Input: part model. Units: mm. Frame: model coordinates. Face numbers are marked on the shaded views. Give positions to 0.01 mm unless a question says otherwise; leave off trailing zeros. Loops run counter-clockwise (first coordinate to the right, second up) from the corner with the lowest first, then second, coordinate; pieces in that order, holes last. Notation, with made-up numbers: (35, 72) -> (81, 72) arc R31 cw to (81, 103) -> close; hole circle Ø5 at (73, 74). An arc over 180 degrees is marked (long way). One line per question, with ' | ' between items.
Autodesk Inventor part; units mm, degrees
ref_plane "Work Plane8" through (0, 0, 20) normal (0, 0, 1) x (1, 0, 0)
ref_plane "YZ Plane" through (0, 0, 0) normal (1, 0, 0) x (0, 1, 0)
ref_plane "XZ Plane" through (0, 0, 0) normal (0, 1, 0) x (-1, 0, 0)
sketch "Sketch1" plane through (0, 0, 0) normal (0, 0, 1) x (1, 0, 0)
  circle A0 centre (0, 0) radius 59.2469 construction
  line L0 (0, 0) -> (59.2469, 0)
  line L1 (0, 0) -> (59.2469, 4.025)
  line L2 (59.2469, 0) -> (59.2469, 4.025)
  circle A1 centre (0, 0) radius 75
  point P0 (56.8, 0)
  dimension "d56" = 59.2469
  dimension "d57" = 4.025
  dimension "d400" = 75
  dimension "d495" = 2.5
  dimension "d496" = 8
  dimension "d531" = 5.5
  dimension "d532" = 5.5
  dimension "d533" = 5.5
  dimension "d537" = 24.5
  dimension "d538" = 3
  dimension "d543" = 5.5
  dimension "d549" = 3
  dimension "d550" = 3
  dimension "d567" = 5.5
  dimension "d568" = 5.5
sketch "Sketch7" plane through (0, 0, 0) normal (0, 1, 0) x (-1, 0, 0)
  line L0 (0, 0) -> (0, 61.9844)
  line L1 (0, 0) -> (-59.2469, 0) construction
  line L2 (0, 61.9844) -> (-59.2469, 0) construction
  line L3 (0, 61.9844) -> (-64.8494, 0) construction
  line L4 (0, 61.9844) -> (-58.9939, -5.5968) construction
  line L5 (0, 0) -> (0, -61.9844)
  line L6 (0, -61.9844) -> (-59.2469, 0) construction
  line L7 (0, -61.9844) -> (-64.8494, 0) construction
  line L8 (0, -61.9844) -> (-58.9939, 5.5968) construction
  line L9 (-58.9939, 5.5968) -> (-64.8494, 0) construction
  line L10 (-54.1083, 0) -> (-62.8579, -8.363) construction
  line L11 (-54.1083, 0) -> (-38.773, -14.6579) construction
  line L12 (0, -94.3812) -> (0, 132.3969)
  line L13 (-75, -5.9919) -> (-75, 6.008)
  line L14 (105, 0) -> (-105, 0)
  line L15 (-62.0481, 2.6775) -> (-56.4456, -2.6775) construction
  line L16 (-56.4456, 2.6775) -> (-62.0481, -2.6775) construction
  line L17 (-26.151, -15.9303) -> (-40.3783, -15.9303) construction
  line L18 (-40.3783, -15.9303) -> (-40.3783, -12.7539) construction
  line L19 (-40.3783, -12.7539) -> (-26.151, -12.7539) construction
  line L20 (-26.151, -12.7539) -> (-26.151, -15.9303) construction
  point P0 (-75, 0)
  dimension "Roller_Side_difference" = -0.0002
  dimension "d90" = 61.9844
  dimension "d201" = 75
  dimension "d343" = 92.587
  dimension "d344" = 92.588
  dimension "d367" = 8.1
sketch "Roller1" plane through (0, 0, 0) normal (0, 1, 0) x (-1, 0, 0)
  line L0 (0, 61.9844) -> (-58.9939, -5.5968) construction
  line L1 (0, 61.9844) -> (-64.8494, 0) construction
  line L2 (-54.1083, 0) -> (-38.773, -14.6579) construction
  line L3 (0, -61.9844) -> (-64.8494, 0) construction
  line L4 (-54.0606, 0.0927) -> (-58.9462, -5.5041)
  line L5 (-58.9462, -5.5041) -> (-64.7589, 0.0519)
  line L6 (-64.7589, 0.0519) -> (-59.3884, 5.1851)
  line L7 (-59.3884, 5.1851) -> (-54.0606, 0.0927)
  line L8 (-56.0019, 1.9482) -> (-61.1299, -3.4168)
  line L9 (-61.8526, -2.7261) -> (-56.7246, 2.639)
  point P0 (0, 0)
  dimension "d345" = 0.025
  dimension "d346" = 0.025
  dimension "d347" = 0.1
  dimension "d348" = 0.1
  dimension "d349" = 272.588
  dimension "d350" = 272.587
  dimension "d617" = 0.9997
sketch "Roller2" plane through (0, 0, 0) normal (0, 1, 0) x (-1, 0, 0)
  line L0 (0, -61.9844) -> (-58.9939, 5.5968) construction
  line L1 (-54.1083, 0) -> (-62.8579, -8.363) construction
  line L2 (0, -61.9844) -> (-64.8494, 0) construction
  line L3 (0, 61.9844) -> (-64.8494, 0) construction
  line L4 (-58.9956, 5.5606) -> (-54.1429, 0.0016)
  line L5 (-54.1429, 0.0016) -> (-59.4789, -5.0987)
  line L6 (-59.4789, -5.0987) -> (-64.8132, 0)
  line L7 (-64.8132, 0) -> (-58.9956, 5.5606)
  line L8 (-61.9044, 2.7803) -> (-56.8109, -2.5486)
  line L9 (-61.1815, 3.4713) -> (-56.088, -1.8576)
  point P0 (0, 0)
  dimension "d351" = 0.025
  dimension "d352" = 0.025
  dimension "d354" = 0.025
  dimension "d355" = 92.587
  dimension "d356" = 92.588
  dimension "d370" = 0.025
  dimension "d371" = 1
sketch "Sketch22" plane through (0, 0, 0) normal (0, 1, 0) x (-1, 0, 0)
  line L0 (-31.756, 8.0215) -> (-17.5287, 8.0215) construction
  line L1 (-17.5287, 8.0215) -> (-17.5287, 4.8451) construction
  line L2 (-17.5287, 4.8451) -> (-31.756, 4.8451) construction
  line L3 (-31.756, 4.8451) -> (-31.756, 8.0215) construction
  point P0 (0, 0)
  dimension "Roller_Side_difference" = -0.0002
sketch "Sketch2" plane through (0, 0, 0) normal (0, 1, 0) x (-1, 0, 0)
  line L0 (0, 0) -> (0, 59.2469) construction
  line L1 (0, 0) -> (-59.2469, 0)
  line L2 (0, 0) -> (0, -59.2469)
  line L3 (0, -59.2469) -> (-59.2469, 0) construction
  line L4 (0, 59.2469) -> (-59.2469, 0) construction
  line L5 (-50.4879, 53.555) -> (0, 59.2469) construction
  line L6 (-29.7354, 7.189) -> (0, 59.2469) construction
  line L7 (-29.7354, 7.189) -> (0, -59.2469) construction
  line L8 (-48.8381, -26.254) -> (0, -59.2469) construction
  point P0 (-40.4258, 18.8211)
sketch "Sketch23" plane through (0, 0, 0) normal (0, 1, 0) x (-1, 0, 0)
  line L0 (0, -61.9844) -> (-58.9939, 5.5968) construction
  line L1 (0, -61.9844) -> (-64.8494, 0) construction
  line L2 (0, 61.9844) -> (-58.9939, -5.5968) construction
  line L3 (-58.9939, 5.5968) -> (-64.8494, 0) construction
  line L4 (0, 61.9844) -> (-64.8494, 0) construction
  line L5 (-58.9939, 5.5968) -> (-58.9939, -5.5968) construction
  line L6 (105, 0) -> (-105, 0)
  line L7 (-57.6514, 4.0968) -> (-54.1326, 0.0658)
  line L8 (-54.1326, -0.0658) -> (-57.6514, -4.0968)
  line L9 (-60.5995, 4.0968) -> (-64.81, 0.0723)
  line L10 (-64.81, -0.0723) -> (-60.5995, -4.0968)
  arc A0 (-64.81, 0.0723) -> (-64.81, -0.0723) centre (-64.7409, 0) ccw
  arc A1 (-54.1326, -0.0658) -> (-54.1326, 0.0658) centre (-54.2079, 0) ccw
  line L11 (-57.6514, 4.0968) -> (-57.6514, 5.5968)
  line L12 (-57.6514, 5.5968) -> (-25, 5.5968)
  line L13 (-25, 5.5968) -> (-25, -5.5968)
  line L14 (-25, -5.5968) -> (-57.6514, -5.5968)
  line L15 (-57.6514, -5.5968) -> (-57.6514, -4.0968)
  line L16 (-60.5995, 4.0968) -> (-60.5995, 5.5968)
  line L17 (-60.5995, 5.5968) -> (-75, 5.5968)
  line L18 (-75, 5.5968) -> (-75, -5.5968)
  line L19 (-60.5995, -4.0968) -> (-60.5995, -5.5968)
  line L20 (-60.5995, -5.5968) -> (-75, -5.5968)
  line L21 (-58.9939, 5.5968) -> (-58.9939, 5.5968)
  line L22 (-58.9939, -5.5968) -> (-58.9939, -5.5968)
  line L23 (0, -94.3812) -> (0, 132.3969)
  line L24 (-64.8856, 0) -> (-75, 0)
  point P0 (0, 0)
  point P1 (-54.0752, 0)
  point P2 (-64.8409, 0)
  point P3 (-75, 0)
  dimension "d378" = 90
  dimension "d379" = 0.1
  dimension "d380" = 0.025
  dimension "d381" = 0.025
  dimension "d382" = 0.025
  dimension "d383" = 0.025
  dimension "d384" = 11.1935
  dimension "d385" = 0
  dimension "d386" = 0
  dimension "d391" = 25
  dimension "d392" = 75
  dimension "d393" = 1.5
  dimension "d394" = 1.5
  dimension "d395" = 1.5
  dimension "d396" = 1.5
revolve "RevRoller1" [suppressed]
fillet "Fillet1" [suppressed]
sketch "Sketch48" plane through (56.7246, 0, 2.639) normal (-0.691, 0, 0.7229) x (0.7229, 0, 0.691)
  line L0 (-2.5, 0.25) -> (2.5, 0.25)
  line L1 (2.5, 0.25) -> (2.5, -0.25)
  line L2 (2.5, -0.25) -> (-2.5, -0.25)
  line L3 (-2.5, -0.25) -> (-2.5, 0.25)
  line L4 (-2.5, 0.25) -> (2.5, -0.25) construction
  line L5 (2.5, 0.25) -> (-2.5, -0.25) construction
  line L6 (-0.25, -2.5) -> (0.25, -2.5)
  line L7 (0.25, -2.5) -> (0.25, 2.5)
  line L8 (0.25, 2.5) -> (-0.25, 2.5)
  line L9 (-0.25, 2.5) -> (-0.25, -2.5)
  line L10 (-0.25, -2.5) -> (0.25, 2.5) construction
  line L11 (0.25, -2.5) -> (-0.25, 2.5) construction
  point P0 (-42.8293, 0)
  point P1 (0, 0)
  point P2 (-0.25, 0.25)
  point P3 (-0.25, -0.25)
  point P4 (0.25, -0.25)
  point P5 (0.25, 0.25)
  dimension "d621" = 5
  dimension "d622" = 0.5
  dimension "d623" = 0.5
  dimension "d624" = 5
extrude "Extrusion39" [suppressed]
sketch "Sketch40" plane through (0, 0, -5.231) normal (0, 0, -1) x (-1, 0, 0)
  circle A0 centre (53.5, 0) radius 2.75
  circle A1 centre (0, 0) radius 53.5
  point P0 (53.4293, 2.7491)
  point P1 (53.4293, -2.7491)
  dimension "d585" = 8
  dimension "d587" = 1.75
  dimension "d589" = 3
  dimension "d592" = 2
  dimension "d593" = 12
  dimension "d594" = 12
  dimension "d611" = 360
pattern_circular "Circular Pattern13" [suppressed]
feature "Move Body7" [suppressed]
revolve "Revolution13" [suppressed]
fillet "Fillet3" [suppressed]
pattern_circular "Circular Pattern14" [suppressed]
feature "Move Body6" [suppressed]
revolve "Revolution14" add sketch "Sketch23" angle 360 about axis through (0, 0, -10) along (0, 0, 1) contours A1 L7 L11 L12 L13 L6 | L6 L13 L14 L15 L8 A1
revolve "OuterRim_Top2" [suppressed]
revolve "OuterRim_Bottom2" [suppressed]
ref_plane "Work Plane8" through (0, 0, 20) normal (0, 0, 1) x (1, 0, 0)
sketch "Sketch49" plane through (0, 0, 20) normal (0, 0, 1) x (1, 0, 0)
  circle A0 centre (0, 0) radius 75
  circle A1 centre (0, 0) radius 60.5995
  circle A2 centre (0, 0) radius 57.6514
  circle A3 centre (0, 0) radius 25
  circle A4 centre (0, 0) radius 69
  circle A5 centre (0, 0) radius 36.75
  point P0 (0, 69)
  point P1 (0, 36.75)
  point P2 (-40.5572, 55.8222)
  dimension "d629" = 69
  dimension "d630" = 73.5
  dimension "d649" = 36
sketch "Sketch50" plane through (0, 0, 5.5968) normal (0, 0, 1) x (1, 0, 0)
  point P0 (0, 0)
  point P1 (0, 69)
sketch "Sketch51" plane through (0, 0, -5.5968) normal (0, 0, -1) x (-1, 0, 0)
  circle A0 centre (0, 0) radius 75
  circle A1 centre (0, 69) radius 2.75
  circle A2 centre (0, 69) radius 1.5
  circle A3 centre (-40.5572, 55.8222) radius 3.5
  circle A4 centre (-40.5572, 55.8222) radius 2
  dimension "d633" = 36
  dimension "d635" = 5.5
  dimension "d636" = 3
  dimension "d637" = 7
  dimension "d638" = 4
extrude "Extrusion40" [suppressed]
extrude "Extrusion41" [suppressed]
extrude "Extrusion42" [suppressed]
extrude "Extrusion43" [suppressed]
sketch "Sketch52" plane through (0, 0, 5.5968) normal (0, 0, 1) x (1, 0, 0)
  circle A0 centre (0, 69) radius 1.5
  circle A1 centre (-40.5572, 55.8222) radius 2
  line L0 (2.75, 67.4123) -> (0, 65.8246)
  line L1 (0, 65.8246) -> (-2.75, 67.4123)
  line L2 (-2.75, 67.4123) -> (-2.75, 70.5877)
  line L3 (-2.75, 70.5877) -> (0, 72.1754)
  line L4 (0, 72.1754) -> (2.75, 70.5877)
  line L5 (2.75, 70.5877) -> (2.75, 67.4123)
  circle A2 centre (0, 0) radius 75
  line L6 (-39.2656, 58.7231) -> (-37.3992, 56.1541)
  line L7 (-36.5379, 56.2446) -> (-38.1817, 52.5526)
  line L8 (-38.1817, 52.5526) -> (-42.201, 52.1301)
  line L9 (-42.201, 52.1301) -> (-44.5765, 55.3997)
  line L10 (-44.5765, 55.3997) -> (-42.9327, 59.0918)
  line L11 (-42.9327, 59.0918) -> (-38.9134, 59.5142)
  line L12 (-38.9134, 59.5142) -> (-36.5379, 56.2446)
  dimension "d651" = 3
  dimension "d652" = 4
  dimension "d655" = 36
  dimension "d657" = 7
  dimension "d658" = 5.5
extrude "Extrusion44" [suppressed]
extrude "Extrusion45" [suppressed]
extrude "Extrusion46" [suppressed]
extrude "Extrusion47" [suppressed]
pattern_circular "Circular Pattern32" [suppressed]
pattern_circular "Circular Pattern33" [suppressed]
sketch "Sketch57" plane through (0, 0, -5.5968) normal (0, 0, -1) x (-1, 0, 0)
  line L0 (-3.175, 39.925) -> (3.175, 39.925)
  line L1 (3.175, 39.925) -> (3.175, 33.575)
  line L2 (3.175, 33.575) -> (-3.175, 33.575)
  line L3 (-3.175, 33.575) -> (-3.175, 39.925)
  line L4 (-3.175, 39.925) -> (3.175, 33.575) construction
  line L5 (3.175, 39.925) -> (-3.175, 33.575) construction
  ellipse E0 centre (0, 36.75) end of major axis (6.4, 36.75) minor radius 5.45
  point P0 (0, 0)
  dimension "d694" = 6.35
  dimension "d695" = 6.35
  dimension "d696" = 6.4
  dimension "d697" = 5.45
extrude "Extrusion50" cut sketch "Sketch57" against normal blind 11.194 contours L0 L1 L2 L3
extrude "Extrusion51" cut sketch "Sketch57" against normal blind 8.194 contours L0 L1 L2 L3 | E0
pattern_circular "Circular Pattern34" count 6 over 360 about axis through (0, 0, -4.8468) along (0, 0, 1) of "Extrusion50", "Extrusion51"
ref_plane "Work Plane9" through (0, 0, -25) normal (0, 0, 1) x (1, 0, 0)
sketch "Sketch58" plane through (0, 0, -25) normal (0, 0, 1) x (1, 0, 0)
  line L0 (0, 0) -> (0, 94.5267)
  line L1 (0, 94.5267) -> (0, 0)
  line L2 (0, 0) -> (-27.705, 103.3964)
  line L3 (0, 0) -> (25.7729, 96.1857)
  circle A0 centre (0, 0) radius 95.9893
  point P0 (-24.8439, 92.7185)
  point P1 (24.8439, 92.7185)
  dimension "d706" = 15
  dimension "d707" = 15
extrude "Extrusion52" cut sketch "Sketch58" along normal through all contours L3 A0 L2 picked at (37.9953, -51.2872)
equation "\"Roller_Side_difference\" = -0.000942deg"
equation "\"Cycloid_Top_Plate_Fasner_Inner\" = 61.25"
equation "\"Cycloid_Top_Plate_Fasner_Outer\" = 85.75"
equation "\"Roller_Hole_Radius\" = 1"
equation "\"Distance_To_Bearing\" = 85.74529"
equation "\"d514\" = 0.2"
equation "\"Machine_Screw_4mm_Head_Dept\" = 4"
equation "\"Machine_Screw_4mm_Head_Diameter\" = 7"
equation "\"Machine_Screw_4mm_HexNut_Thickness\" = 3"
equation "\"Machine_Screw_4mm_HexNut_Width\" = 6.9"
equation "\"Machine_Screw_4mm_Length\" = 8"
equation "\"Fastner_4mm_Hex_Nut_Width\" = 7"
equation "\"Fastner_4mm_Screw_Diameter\" = 4"
equation "\"Fastner_4mm_Screw_Head_Diameter\" = 7"
equation "\"Fastner_4mm_Hex_Nut_Hole_Dept\" = 3.19352"
equation "\"Fastner_4mm_Screw_Head_Hole_Dept\" = 4"
properties part number "Section_Left_OuterBearing_TBS"
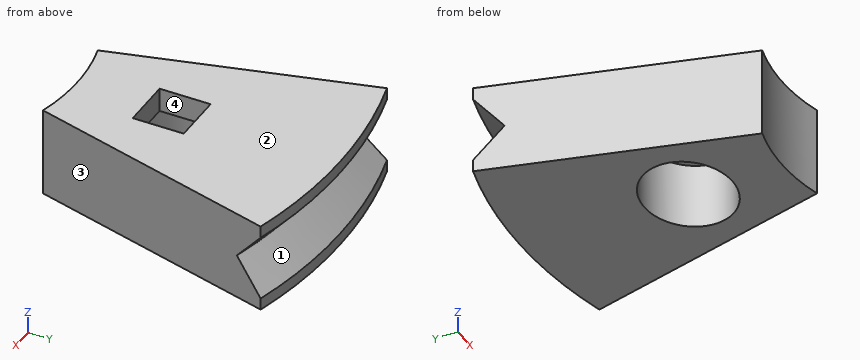
1. Section query B-B (y = 46). Output: boundary loops of the cut face in (x, z).
Determined:
outline: (-12.33, -5.6) -> (12.33, -5.6) -> (12.33, 5.6) -> (-12.33, 5.6) -> close
2. Ray query, line 1 along Z through (x, y) = (-0.25, 33); line 2 along Y through (x, z) = (1, -3.25); line 3 along X through (y, z) = (46, 1). Return the intervals inside material, ascending. Write a range as from..to.
Determined:
line 1: z = 2.6..5.6 | line 2: y = 24.98..31.37, 42.13..56.9 | line 3: x = -12.33..12.33
3. Section query A-A (z = 3). Output: boundary loops of the cut face in (x, y) (3 decimals).
Determined:
outline: (-14.673, 54.762) -> (-6.47, 24.148) arc R25 cw to (6.47, 24.148) -> (14.673, 54.762) arc R56.694 ccw to start; hole (-3.175, 33.575) -> (3.175, 33.575) -> (3.175, 39.925) -> (-3.175, 39.925) -> close
4. Pull-direction query (Y, two-part tool) for the marked faces 1, 2, 3 and 4; classes: pulls with the +Y half, pulls with the -Y half, needs draft (parallel to the pull), parting line crosses it, or undercut.
Determined:
face 1: pulls with the +Y half | face 2: needs draft | face 3: pulls with the -Y half | face 4: undercut
5. Pin query (flat end, axial travel): P1, Ø2.5, axis at y = 36.5, z = 3.5, coming from the +X side; P2, Ø2.5, axis at y = 37, z = 4.5, coming from the -X side; P3, Ø1.5, axis at x = 1.5, z = 4.5, coming from the -Y side. Return the tip coordinate at first contact, or that it passes through.
Determined:
P1: stops at x = 10.12 | P2: stops at x = -10.25 | P3: stops at y = 24.9
